```python
from build123d import *

# Parameters (mm, degrees)
F1_DEPTH  = 25.4
F2_R      = 6.604
F3_DEPTH  = 101.601
F4_R      = 13.97
F5_DEPTH  = 12.7
F6_R      = 6.604
F7_DEPTH  = 101.601
F8_R      = 13.97
F9_DEPTH  = 12.7
F10_R     = 6.604
F11_DEPTH = 101.601
F12_R     = 13.97
F13_DEPTH = 12.7
F14_R     = 6.604
F15_DEPTH = 101.601
F16_R     = 13.97
F17_DEPTH = 12.7


with BuildPart() as f1:
    # F0 (on Front) → F1 (new body, symmetric)
    with BuildSketch(Plane.XZ):
        with BuildLine():
            ThreePointArc((127.27204, -151.351064), (-12.964423, -207.50014), (-153.200886, -151.351064))
            Line((-153.200886, -151.351064), (-216.700886, -151.351064))
            Line((-216.700886, -151.351064), (-216.700886, -252.951064))
            Line((-216.700886, -252.951064), (1002.499114, -252.951064))
            Line((1002.499114, -252.951064), (1002.499114, -151.351064))
            Line((1002.499114, -151.351064), (938.999114, -151.351064))
            ThreePointArc((938.999114, -151.351064), (794.496976, -211.689691), (649.994838, -151.351064))
            Line((649.994838, -151.351064), (535.694838, -151.351064))
            ThreePointArc((535.694838, -151.351064), (388.633439, -214.325586), (241.57204, -151.351064))
            Line((241.57204, -151.351064), (127.27204, -151.351064))
        make_face()
    extrude(amount=F1_DEPTH, both=True)

    # F2 (on face) → F3 (cut, through all)
    with BuildSketch(Plane.XY.offset(-151.351064)):
        with Locations((-184.950886, 0)):
            Circle(F2_R)
    extrude(amount=-F3_DEPTH, mode=Mode.SUBTRACT)

    # F4 (on face) → F5 (cut)
    with BuildSketch(Plane.XY.offset(-151.351064)):
        with Locations((-184.950886, 0)):
            Circle(F4_R)
    extrude(amount=-F5_DEPTH, mode=Mode.SUBTRACT)

    # F6 (on face) → F7 (cut, through all)
    with BuildSketch(Plane.XY.offset(-151.351064)):
        with Locations((184.42204, 0)):
            Circle(F6_R)
    extrude(amount=-F7_DEPTH, mode=Mode.SUBTRACT)

    # F8 (on face) → F9 (cut)
    with BuildSketch(Plane.XY.offset(-151.351064)):
        with Locations((184.42204, 0)):
            Circle(F8_R)
    extrude(amount=-F9_DEPTH, mode=Mode.SUBTRACT)

    # F10 (on face) → F11 (cut, through all)
    with BuildSketch(Plane.XY.offset(-151.351064)):
        with Locations((592.844838, 0)):
            Circle(F10_R)
    extrude(amount=-F11_DEPTH, mode=Mode.SUBTRACT)

    # F12 (on face) → F13 (cut)
    with BuildSketch(Plane.XY.offset(-151.351064)):
        with Locations((592.844838, 0)):
            Circle(F12_R)
    extrude(amount=-F13_DEPTH, mode=Mode.SUBTRACT)

    # F14 (on face) → F15 (cut, through all)
    with BuildSketch(Plane.XY.offset(-151.351064)):
        with Locations((970.749114, 0)):
            Circle(F14_R)
    extrude(amount=-F15_DEPTH, mode=Mode.SUBTRACT)

    # F16 (on face) → F17 (cut)
    with BuildSketch(Plane.XY.offset(-151.351064)):
        with Locations((970.749114, 0)):
            Circle(F16_R)
    extrude(amount=-F17_DEPTH, mode=Mode.SUBTRACT)


solid = f1.part
```
Can you work these out from the model? Positions are in its coordinate system, mm. A direction names the side the tool comes from. Coordinates: 2 decimals unless noted, no trailing zeros. Loops run counter-clockwise (first coordinate to the right, second up) from the corner with the lowest first, then second, coordinate; pieces in that order, holes last. Notation, with made-up numbers: M 33,42.5 L 66,42.5 A15 cw 66,66.5 Z; hole C 60.5,1 d3. An arc over 180 degrees is marked long. Put each result on its own line as item: value. Start each with the question number.
(1) Imagine slicing it at B-B on x = 801. List the corners of the cut face in (y, z) for me, and give its area (3 significant figures).
(2) Which directions (+Z, -Z, +X, -X, +Y, -Y) give clear straight access to the entire face, cutting with the end or side of a thin tool? Please do faces 4 (the face through (596, -6, -164.051)), 5 (the face through (796.747, -0.356, -211.677)).
(3) We'd pull the mould along X, two halves only. Please class faces 1 (the face through (606.3, 5.3, -151.351)), 2 (the face through (1002.499, 0, -203)), 3 (the face through (-195.25, 9.44, -157.61)): +X half, -X half, draft (parallel to the pull), parting line (faces both ways), or undercut.
(4) Imagine slicing it at A-A on x = 87.5. List the corners of the cut face in (y, z) for me, and give its area (3 significant figures).
(5) Will these pins go through, and if not, where does the flat tip stop? pin 1 Ø17 at (x, y) = (592.84, 0) entering from +Z; pin 2 Ø12 at (x, y) = (184.42, 0) entering from -Z.
(6) I need wall thicknesses on probe 1 along X at (y, z) = (-19.5, -179); probe 2 along X at (y, z) = (22.5, -181); probe 3 along X at (y, z) = (-2.5, -217). Which ranges of each line are inside material? Lowest first, please.
Worked answers:
1. outline: M -25.4,-252.95 L 25.4,-252.95 L 25.4,-211.59 L -25.4,-211.59 Z
1. area: 2,100 mm2
2. face 4: +Z
2. face 5: +Z, +Y, -Y
3. face 1: draft
3. face 2: +X half
3. face 3: undercut
4. outline: M -25.4,-252.95 L 25.4,-252.95 L 25.4,-180.93 L -25.4,-180.93 Z
4. area: 3,660 mm2
5. pin 1: stops at z = -164.05
5. pin 2: passes through
6. probe 1: x = -216.7 to -116.74, 90.82 to 274.14, 503.13 to 683.97, 905.03 to 1002.5
6. probe 2: x = -216.7 to -113.3, 87.37 to 277.13, 500.14 to 687.12, 901.88 to 1002.5
6. probe 3: x = -216.7 to -191.06, -178.84 to 178.31, 190.53 to 586.73, 598.96 to 964.64, 976.86 to 1002.5
